Geometry check sheet. Reference: drawing and pictorial views, mm from the part's lowest x, y, z. A direction names the side the tool comes from. Give positions to 0.01 mm unless a question says otherwise; leave off trailing zeros. Order: outer loops, then holes, each group sorted by start corner. A loop starts at its lowest first (then second) coordinate and runs counter-clockwise, first axis right, second up.
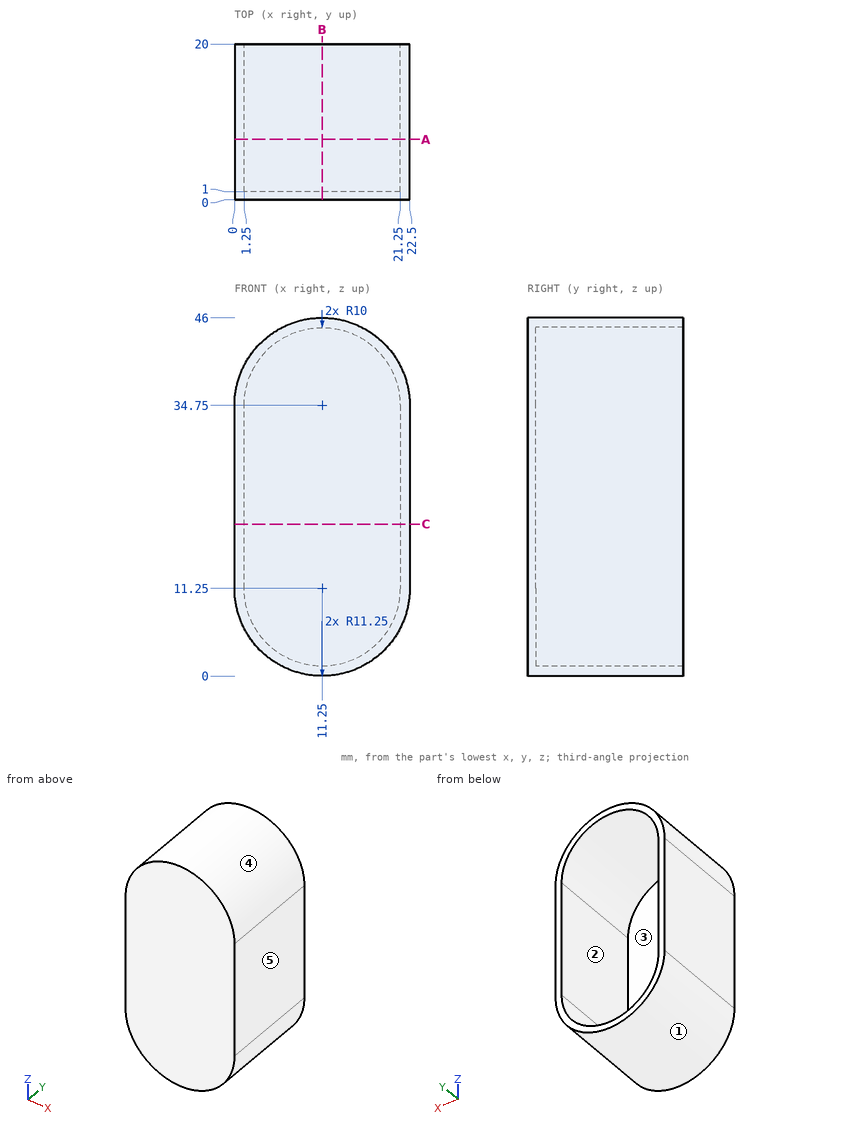
(1) Release check for a two-part mould opening along X. For the marked faces 3, 4 and 5 record: released by +X, released by -X, zero draft, split by the parting line, or undercut.
Response values:
face 3: undercut
face 4: split by the parting line
face 5: released by +X
(2) Cross-section at B-B on x = 11.25. Enter the section's corners in (y, z), then the cut area to 3 significant figures.
Response values:
outline: (0, 0) - (20, 0) - (20, 1.25) - (1, 1.25) - (1, 44.75) - (20, 44.75) - (20, 46) - (0, 46) - close
area: 93.5 mm2
(3) Gauge pin test, flat ends, axial feed: pin 1 Ø2 at (y, z) = (15, 4.5) entering from +X; pin 2 Ø1.5 at (x, y) = (16, 6.5) entering from -Z; pin 3 Ø5 at (x, y) = (17, 4.5) entering from -Z. Record the tip position at first contact, or that the pin passes through.
Response values:
pin 1: stops at x = 20.92
pin 2: stops at z = 0.74
pin 3: stops at z = 0.48
(4) Set-up check for the marked faces 1 and 2: record each of +Z, -Z, +X, -X, +Y, -Y from which the full face is reachable in a straight line by a thin tool's end or side.
Response values:
face 1: -Z, +Y, -Y
face 2: +Y
(5) Cross-section at A-A on y = 7.75. Enter the section's corners in (x, z).
Response values:
outline: (0, 11.25) arc R11.25 ccw to (22.5, 11.25) - (22.5, 34.75) arc R11.25 ccw to (0, 34.75) - close; hole (1.25, 11.25) arc R10 ccw to (21.25, 11.25) - (21.25, 34.75) arc R10 ccw to (1.25, 34.75) - close
(6) Cross-section at C-C on z = 19.5. Enter the section's corners in (x, y).
Response values:
outline: (0, 0) - (22.5, 0) - (22.5, 20) - (21.25, 20) - (21.25, 1) - (1.25, 1) - (1.25, 20) - (0, 20) - close
(7) Material ranges on L1, parallel to X at y = 6.25, z = 25; L2, parallel to Y at x = 5, z = 35.5; L3, parallel to Z at x = 14, y = 10, recorded low to high.
Response values:
L1: x = 0 to 1.25, 21.25 to 22.5
L2: y = 0 to 1
L3: z = 0.34 to 1.64, 44.36 to 45.66
